Input: part model. Units: mm. Frame: model coordinates. A direction names the side the tool comes from. Round coordinates to 2 decimals unless told otherwise and drop trailing zeros. Loops run counter-clockwise (first coordinate to the right, second up) from the corner with the lowest first, then second, coordinate; pieces in that order, holes last.
1) Section A-A, the plane y = 0.2. Return loops of the section in (x, z), and give its area (3 significant figures).
2) Draft query along Z for faces 1 (the face through (1.5, 0.5, 0)), 2 (the face through (1, 1, -25)), 3 (the face through (0.5, 0.5, -48)). Return one class per face: pulls with the +Z half, pulls with the -Z half, needs draft (parallel to the pull), parting line crosses it, or undercut.
3) Access query for faces 4 (the face through (1.5, 0.5, -50)), 5 (the face through (2.5, 0.5, -2)). Directions: +Z, -Z, +X, -X, +Y, -Y. A direction counts if a zero-diameter tool reaches every point of the face in a straight line with its end or side. Return the directions, or none.
4) Ray query, line 1 along Z through (x, y) = (0.7, 0.95). Return the intervals inside material, ascending.
5) Section B-B, the plane x = 1.75. Return loops of the section in (y, z).
from build123d import *

# Parameters (mm, degrees)
ESBO_O1_W                = 3
ESBO_O1_H                = 1
RESSALTO_EXTRUS_O1_DEPTH = 50
ESBO_O3_W                = 2
ESBO_O3_H                = 2
CORTE_EXTRUS_O1_DEPTH    = 44


with BuildPart() as part:
    # Esboço1 → Ressalto-extrusão1 (new body)
    with BuildSketch(Plane.XY):
        with Locations((1.5, 0.5)):
            Rectangle(ESBO_O1_W, ESBO_O1_H)
    extrude(amount=-RESSALTO_EXTRUS_O1_DEPTH)

    # Esboço3 → Corte-extrusão1 (cut)
    with BuildSketch(Plane(origin=(0, 1, 0), x_dir=(1, 0, 0), z_dir=(0, 1, 0))):
        with Locations((1.5, 2)):
            Rectangle(ESBO_O3_W, ESBO_O3_H)
        with Locations((1.5, 48)):
            Rectangle(ESBO_O3_W, ESBO_O3_H)
    extrude(amount=-CORTE_EXTRUS_O1_DEPTH, mode=Mode.SUBTRACT)


solid = part.part
Final values:
1. outline: (0, -50) - (3, -50) - (3, 0) - (0, 0) - close; hole (0.5, -49) - (2.5, -49) - (2.5, -47) - (0.5, -47) - close; hole (0.5, -3) - (2.5, -3) - (2.5, -1) - (0.5, -1) - close
1. area: 142 mm2
2. face 1: pulls with the +Z half
2. face 2: needs draft
2. face 3: undercut
3. face 4: -Z, +X, -X, +Y, -Y
3. face 5: +Y, -Y
4. line 1: z = -50 to -49, -47 to -3, -1 to 0
5. outline: (0, -50) - (1, -50) - (1, -49) - (0, -49) - close; (0, -47) - (1, -47) - (1, -3) - (0, -3) - close; (0, -1) - (1, -1) - (1, 0) - (0, 0) - close
